Source: CAD feature listing. Evaluate the final solid. Frame: model axes, mm. A direction names the side the tool comes from. Round coordinates to 2 decimals unless told otherwise and drop trailing zeros. Order: outer loops, then holes, each group sorted by start corner. A loop starts at its lowest first (then second) coordinate and runs counter-clockwise, first axis right, second up. Notation, with made-up numbers: (47.25, -26) - (84.25, -26) arc R20 cw to (84.25, 9) - close; hole circle Ø3 at (50.5, 41.5). An arc over 180 degrees is marked (long way). Use one line per item in the form item = value. Start each with the question number.
Q1. Cut plane D-D, the plane y = 108.5. Return the cut outline in (x, z).
Q2. Set-up query: faces 4 (the flat face through (5, 132, -5)), 5 (the flat face through (-5, 132, -5)), 6 (the cylindrical face through (5.38, 78.43, 4.93)), 7 (the cylindrical face through (-1.08, 105.05, 0.12)). Return all of +Z, -Z, +X, -X, +Y, -Y with unobstructed straight access to the full face (end or side cutting, diameter ignored); none if empty.
Q3. Draft query along Y for faces 1 (the cylindrical face through (189.237, 16.17, 4.93)), 2 (the flat face through (-3, 36, 10)), 3 (the flat face through (99.367, 63.528, 4.93)). Return one class per face: released by +Y, released by -Y, zero draft, split by the parting line, or undercut.
Q4. Cut plane B-B, the plane y = 70. Return the cut outline in (x, z), and give its area (3 significant figures).
Q5. Pin query (flat end, axial travel): pin 1 Ø1.5 at (x, y) = (-45.5, 51) entering from +Z; pin 2 Ø12 at (x, y) = (-180, 20) entering from -Z; pin 3 Ø1 at (x, z) = (-141.5, 3.5) entering from +Y; pin 4 Ø15 at (y, z) = (130, -2) entering from -X. Return the tip coordinate at first contact, or that it passes through.
Q6. Cut plane C-C, the plane x = -130. Return the cut outline in (y, z), and give its area (3 significant figures).
Q7. Ray query, line 1 (Y direction, x = 2, z = 5); line 2 (Y direction, x = 0, z = 3); line 3 (Z direction, x = -92.5, y = 38). Return the intervals inside material, ascending. Write a range as [from, to].
Q8. Cut plane A-A, the plane y = 20. Return the cut outline in (x, z).
from build123d import *

# Parameters (mm, degrees)
SKETCH_1_R           = 10
EXTRUDE_1_DEPTH      = 10
EXTRUDE_START        = -85
SKETCH_2_R           = 5
EXTRUDE_2_DEPTH      = 40
SKETCH_3_R           = 15
SKETCH_3_R_2         = 10
EXTRUDE_3_DEPTH      = 5
EXTRUDE_3_DEPTH_BACK = 5


with BuildPart() as part:
    # Sketch 1 → Extrude 1 (new body)
    with BuildSketch(Plane.XY):
        with BuildLine():
            Line((-10.860669242, 88.497348787), (-185.430334621, 39.248674393))
            ThreePointArc((-185.430334621, 39.248674393), (-199.8112782, 17.258968065), (-180, 0))
            Line((-180, 0), (180, 0))
            ThreePointArc((180, 0), (199.8112782, 17.258968065), (185.430334621, 39.248674393))
            Line((185.430334621, 39.248674393), (10.860669242, 88.497348787))
            ThreePointArc((10.860669242, 88.497348787), (0, 90), (-10.860669242, 88.497348787))
        make_face()
        with Locations((-180, 20)):
            Circle(SKETCH_1_R, mode=Mode.SUBTRACT)
        with Locations((180, 20)):
            Circle(SKETCH_1_R, mode=Mode.SUBTRACT)
        with Locations((0, 70)):
            Circle(SKETCH_1_R, mode=Mode.SUBTRACT)
    extrude(amount=EXTRUDE_1_DEPTH)

    # Sketch 2 → Extrude 2 (add)
    with BuildSketch(Plane.XZ.offset(EXTRUDE_START)):
        with Locations((0, 5)):
            Circle(SKETCH_2_R)
    extrude(amount=-EXTRUDE_2_DEPTH)

    # Sketch 3 → Extrude 3 (add, two sides)
    with BuildSketch(Plane(origin=(0, 0, 0), x_dir=(0, 0, -1), z_dir=(1, 0, 0))) as extrude_3_sk:
        with Locations((-5, 135)):
            Circle(SKETCH_3_R)
        with Locations((-5, 135)):
            Circle(SKETCH_3_R_2, mode=Mode.SUBTRACT)
    extrude(amount=EXTRUDE_3_DEPTH)
    extrude(extrude_3_sk.sketch, amount=-EXTRUDE_3_DEPTH_BACK)


solid = part.part
Completed:
q1.outline = circle Ø10 at (0, 5)
q2.face_4 = +Z, -Z, +X, +Y
q2.face_5 = +Z, -Z, -X, +Y
q2.face_6 = +Z, -Z
q2.face_7 = none
q3.face_1 = undercut
q3.face_2 = zero draft
q3.face_3 = released by +Y
q4.outline = (-76.43, 0) - (-10, 0) - (-10, 10) - (-76.43, 10) - close; (10, 0) - (76.43, 0) - (76.43, 10) - (10, 10) - close
q4.area = 1,330 mm2
q5.pin_1 = 10
q5.pin_2 = through
q5.pin_3 = 51.78
q5.pin_4 = -5
q6.outline = (0, 0) - (54.89, 0) - (54.89, 10) - (0, 10) - close
q6.area = 549 mm2
q7.line_1 = [0, 60.2], [79.8, 125], [145, 150]
q7.line_2 = [0, 60], [80, 125.2], [144.8, 149.87]
q7.line_3 = [0, 10]
q8.outline = (-200, 0) - (-190, 0) - (-190, 10) - (-200, 10) - close; (-170, 0) - (170, 0) - (170, 10) - (-170, 10) - close; (190, 0) - (200, 0) - (200, 10) - (190, 10) - close
